For this review, take the finished solid that the model builds, in its own axes (mm). A direction names the side the tool comes from. Coordinates: 2 decimals unless noted, no trailing zeros. Order: outer loops, then holes, each group sorted by start corner. A loop starts at its lowest first (then second) coordinate and runs counter-clockwise, first axis right, second up.
from build123d import *

# Parameters (mm, degrees)
SKETCH_2_OUTSIDE_W  = 48.8
SKETCH_2_OUTSIDE_H  = 48.8
CUT_EXTRUDE_1_DEPTH = 30


with BuildPart() as part:
    # Эскиз1 → Повернуть1 (revolve)
    with BuildSketch(Plane.XY, mode=Mode.PRIVATE) as revolve_1_sk:
        Polygon((18, 12), (18, 15.401923789), (16.5, 18), (1.5, 18), (0, 15.401923789), (0, 12), (10, 12), (10, 13), (12, 13), (12, 8), (18, 8), align=None)
    revolve(revolve_1_sk.sketch.rotate(Axis((0, 0, 0), (1, 0, 0)), 90), axis=Axis((0, 0, 0), (1, 0, 0)))

    # Эскиз2 outside → Вырез-Вытянуть1 (cut)
    with BuildSketch(Plane(origin=(18, 0, 0), x_dir=(0, 0, -1), z_dir=(1, 0, 0))):
        Rectangle(SKETCH_2_OUTSIDE_W, SKETCH_2_OUTSIDE_H)
        Polygon((0, 18), (-15.588457268, 9), (-15.588457268, -9), (0, -18), (15.588457268, -9), (15.588457268, 9), align=None, mode=Mode.SUBTRACT)
    extrude(amount=-CUT_EXTRUDE_1_DEPTH, mode=Mode.SUBTRACT)


solid = part.part
1. Take a section at A-A, the plane x = 16. Give the boundary of the cut face in (y, z), plus the area to 3 significant figures.
Answer below:
outline: (-18, 0) - (-9, -15.59) - (9, -15.59) - (18, 0) - (9, 15.59) - (-9, 15.59) - close; hole circle Ø16 at (0, 0)
area: 641 mm2
2. Clearance check with flat-ended pins moving along their axes: pin 1 Ø5 at (x, z) = (15.5, 10) entering from +Y; pin 2 Ø6 at (x, z) = (13, 1) entering from -Y; pin 3 Ø2 at (x, y) = (5, 12.5) entering from -Z. State where each tip first meets the part, or that it passes through.
Answer below:
pin 1: stops at y = 13.67
pin 2: stops at y = -18
pin 3: stops at z = -11.26
3. Take a section at B-B, the plane y = 0. Give the boundary of the cut face in (x, z), plus the area to 3 significant figures.
Answer below:
outline: (0, -15.4) - (0.11, -15.59) - (17.89, -15.59) - (18, -15.4) - (18, -8) - (12, -8) - (12, -13) - (10, -13) - (10, -12) - (0, -12) - close; (0, 12) - (10, 12) - (10, 13) - (12, 13) - (12, 8) - (18, 8) - (18, 15.4) - (17.89, 15.59) - (0.11, 15.59) - (0, 15.4) - close
area: 173 mm2
4. To check wall thickness, follow L1, parallel to Y at x = 5, z = -1; L2, parallel to Z at x = 16.75, y = -7; L3, parallel to X at y = 11, z = 4. State the ranges of each line that lie inside material, in increasing order.
Answer below:
L1: y = -17.42 to -11.96, 11.96 to 17.42
L2: z = -15.59 to -3.87, 3.87 to 15.59
L3: x = 12 to 18
5. Take a section at C-C, the plane x = 5.5. Give the boundary of the cut face in (y, z).
Answer below:
outline: (-18, 0) - (-9, -15.59) - (9, -15.59) - (18, 0) - (9, 15.59) - (-9, 15.59) - close; hole circle Ø24 at (0, 0)
6. The part is to be moulded in two halves that separate along X. For faces 1 (the face through (0, 12.5, -0.1)), 2 (the face through (9, 0, 15.588)), 3 (the face through (11.014, 7.91, -10.316)), 4 (the face through (10, 9, -9)), say which applies: +X half, -X half, draft (parallel to the pull), parting line (faces both ways), or undercut.
Answer below:
face 1: -X half
face 2: draft
face 3: undercut
face 4: undercut
7. Machinability: for faces 5 (the face through (9, 0, -15.588)), 6 (the face through (5.07, -3.604, 11.446)), 7 (the face through (12, -6, 6)), which of the approach directions +Z, -Z, +X, -X, +Y, -Y give a long, thin tool a straight path to every point of the face, cutting with its end or side? Answer none if there is none.
Answer below:
face 5: -Z, +X, -X, +Y, -Y
face 6: -X
face 7: none
